Design review of the part built by this model. Coordinates are the model's own, in mm. Face numbers are marked on the shaded views. A direction names the side the tool comes from. Round coordinates to 2 decimals unless told otherwise and drop trailing zeros. Order: outer loops, then holes, each group sorted by start corner. A loop starts at its lowest first (then second) coordinate and runs counter-clockwise, first axis right, second up. Notation, with made-up numbers: (-2.75, 86.5) - (7.25, 86.5) arc R3 cw to (7.25, 91.5) - close; hole circle Ø8 at (-3.75, 21). An arc over 180 degrees is marked (long way). Answer as a JSON object with one key per item and string values. Group by question number.
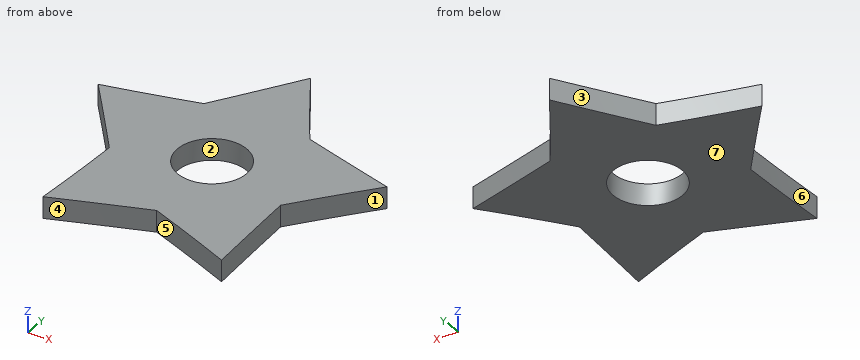
from build123d import *

# Parameters (mm, degrees)
F0_R     = 11.2
F1_DEPTH = 7


with BuildPart() as f1:
    # F0 (on Top) → F1 (new body)
    with BuildSketch(Plane.XY):
        with BuildLine():
            ThreePointArc((0, 48.90934), (-8.622128, 35.760107), (-17.34349, 22.676482))
            ThreePointArc((-17.34349, 22.676482), (-31.889544, 18.740952), (-46.515547, 15.113817))
            ThreePointArc((-46.515547, 15.113817), (-36.674267, 2.85035), (-26.926049, -9.487221))
            ThreePointArc((-26.926049, -9.487221), (-27.678115, -24.537486), (-28.748189, -39.568487))
            ThreePointArc((-28.748189, -39.568487), (-14.043816, -33.998494), (0.702277, -28.539907))
            ThreePointArc((0.702277, -28.539907), (14.783528, -33.905952), (28.748189, -39.568487))
            ThreePointArc((28.748189, -39.568487), (27.994711, -23.862575), (27.36008, -8.151411))
            ThreePointArc((27.36008, -8.151411), (36.814838, 3.582455), (46.515547, 15.113817))
            ThreePointArc((46.515547, 15.113817), (31.345499, 19.250612), (16.207183, 23.502058))
            ThreePointArc((16.207183, 23.502058), (7.969293, 36.120031), (0, 48.90934))
        make_face()
        Circle(F0_R, mode=Mode.SUBTRACT)
    extrude(amount=F1_DEPTH)


solid = f1.part
1. Take a section at B-B, the plane x = 4.5. Give the boundary of the cut face in (y, z).
2. Take a section at C-C, the plane y = 2.5. Give the boundary of the cut face in (x, z), then the cut area to 3 significant figures.
3. Take a section at A-A, the plane z = 5.5. Give the boundary of the cut face in (x, y) (1 decimal).
4. Tool access review of the marked faces 5, 6 and 7: name each direction out of +Z, -Z, +X, -X, +Y, -Y from which nothing blocks a thin tool from reaching the whole face with its end or side.
5. Take a section at D-D, the plane y = -19. Give the boundary of the cut face in (x, z), then the cut area to 3 significant figures.
6. Mouldability with a two-part tool opening along X and no side actions: class the marked faces 1, 2, 3 and 4 as pulls with the +X half, pulls with the -X half, needs draft (parallel to the pull), parting line crosses it, or undercut.
7. To check wall thickness, follow line 1 (Y direction, x = 8, z = 6.25); line 2 (Y direction, x = -1, z = 5.5); line 3 (X direction, y = 8.5, z = 5.25). State the ranges of each line that lie inside material, in increasing order. Write a range as from..to.
8. Clearance check with flat-ended pins moving along their axes: P1, Ø2, axis at y = 36, z = 5.5, coming from the -X side; P2, Ø3, axis at y = 33.5, z = 4, coming from the -X side. State where each tip first meets the part, or that it passes through.
Response values:
{
 "1": {"outline": "(-29.95, 0) - (-10.26, 0) - (-10.26, 7) - (-29.95, 7) - close; (10.26, 0) - (41.61, 0) - (41.61, 7) - (10.26, 7) - close"},
 "2": {"outline": "(-36.4, 0) - (-10.92, 0) - (-10.92, 7) - (-36.4, 7) - close; (10.92, 0) - (35.93, 0) - (35.93, 7) - (10.92, 7) - close", "area": "353 mm2"},
 "3": {"outline": "(-46.5, 15.1) arc R2078.3 cw to (-26.9, -9.5) arc R712.8 cw to (-28.7, -39.6) arc R2078.3 cw to (0.7, -28.5) arc R712.8 cw to (28.7, -39.6) arc R2078.3 cw to (27.4, -8.2) arc R712.8 cw to (46.5, 15.1) arc R2078.4 cw to (16.2, 23.5) arc R712.8 cw to (0, 48.9) arc R2078.4 cw to (-17.3, 22.7) arc R712.8 cw to start; hole circle Ø22.4 at (0, 0)"},
 "4": {"face 5": "+Z, -Z, -Y", "face 6": "+Z, -Z, -X", "face 7": "-Z, +X, -X, +Y, -Y"},
 "5": {"outline": "(-27.36, 0) - (27.79, 0) - (27.79, 7) - (-27.36, 7) - close", "area": "386 mm2"},
 "6": {"face 1": "pulls with the +X half", "face 2": "undercut", "face 3": "pulls with the -X half", "face 4": "undercut"},
 "7": {"line 1": "-31.28..-7.84, 7.84..36.07", "line 2": "-29.16..-11.16, 11.16..47.37", "line 3": "-41.19..-7.29, 7.29..40.9"},
 "8": {"P1": "x = -9.12", "P2": "x = -11.11"}
}
